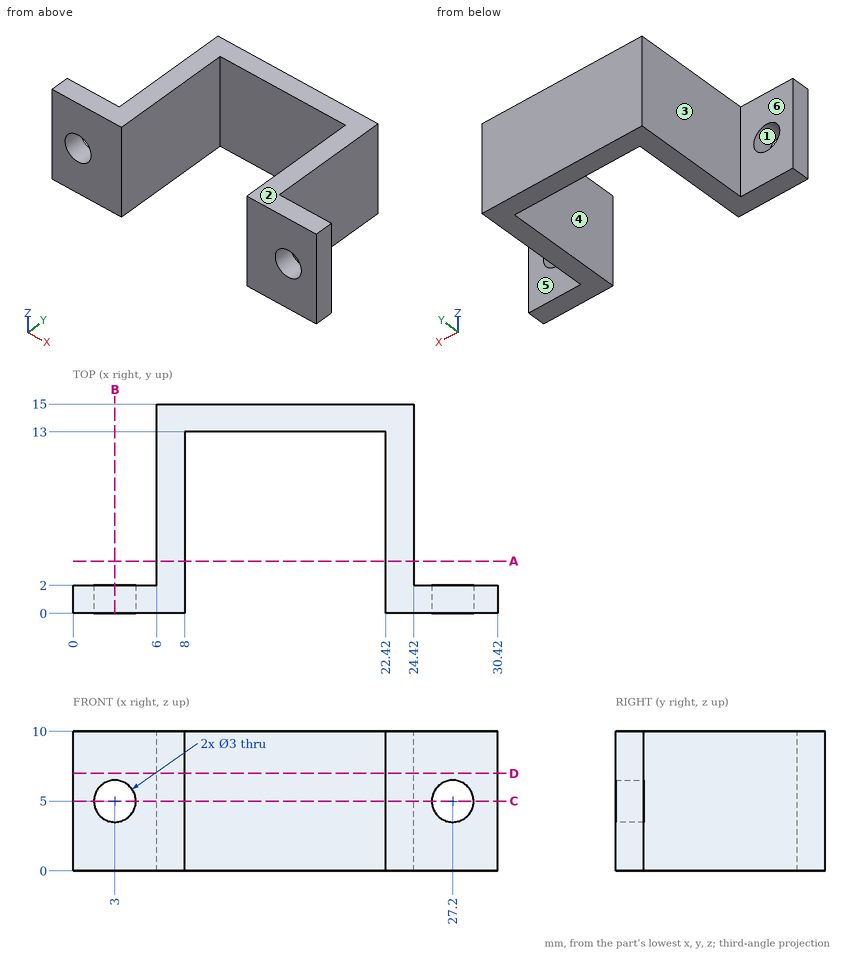
Part print with two shaded views. Sizes in mm from the minimum x, y, z corner. A direction names the side the tool comes from. Coordinates: 2 decimals unless noted, no trailing zeros. Order: outer loops, then holes, each group sorted by start corner. A loop starts at its lowest first (then second) coordinate and runs counter-clockwise, first axis right, second up.
(1) Pin check, flat tips, straight feed: pin 1 Ø1.8 at (x, z) = (3, 3) entering from +Y; pin 2 Ø5 at (y, z) = (8.5, 6.5) entering from -X; pin 3 Ø3 at (y, z) = (4, 3.5) entering from +X. Stop position of each tip, or through.
Solution:
pin 1: stops at y = 2
pin 2: stops at x = 6
pin 3: stops at x = 24.42
(2) Mould opens along Z. For the marked faces 1, 2 and 3 say: released by +Z, released by -Z, zero draft, split by the parting line, or undercut.
Solution:
face 1: undercut
face 2: released by +Z
face 3: zero draft
(3) Saw through at A-A, the plane y = 3.75. Write the cut outline in (x, z), and give its area (3 significant figures).
Solution:
outline: (6, 0) - (8, 0) - (8, 10) - (6, 10) - close; (22.42, 0) - (24.42, 0) - (24.42, 10) - (22.42, 10) - close
area: 40.0 mm2
(4) Saw through at B-B, the plane x = 3. Write the cut outline in (y, z).
Solution:
outline: (0, 0) - (2, 0) - (2, 3.5) - (0, 3.5) - close; (0, 6.5) - (2, 6.5) - (2, 10) - (0, 10) - close
(5) Saw through at D-D, the plane z = 7. Write the cut outline in (x, y), and give its area (3 significant figures).
Solution:
outline: (0, 0) - (8, 0) - (8, 13) - (22.42, 13) - (22.42, 0) - (30.42, 0) - (30.42, 2) - (24.42, 2) - (24.42, 15) - (6, 15) - (6, 2) - (0, 2) - close
area: 113 mm2
(6) Saw through at C-C, the plane z = 5. Write the cut outline in (x, y).
Solution:
outline: (0, 0) - (1.5, 0) - (1.5, 2) - (0, 2) - close; (4.5, 0) - (8, 0) - (8, 13) - (22.42, 13) - (22.42, 0) - (25.7, 0) - (25.7, 2) - (24.42, 2) - (24.42, 15) - (6, 15) - (6, 2) - (4.5, 2) - close; (28.7, 0) - (30.42, 0) - (30.42, 2) - (28.7, 2) - close
(7) Which spindle directions (+Z, -Z, +X, -X, +Y, -Y) get a long thin tool onto all of the face, cutting with end or side? Do the marked faces 4, 5 and 6. Say none if no direction does.
Solution:
face 4: +Z, -Z, -Y
face 5: +Z, -Z, +X, +Y
face 6: +Z, -Z, -X, +Y
(8) Drill centre lines: L1, parallel to X at y = 0.6, z = 5; L2, parallel to X at y = 7.5, z = 7.25; L3, parallel to X at y = 1.75, z = 6. Where is each one in solid material? Low to high.
Solution:
L1: x = 0 to 1.5, 4.5 to 8, 22.42 to 25.7, 28.7 to 30.42
L2: x = 6 to 8, 22.42 to 24.42
L3: x = 0 to 1.88, 4.12 to 8, 22.42 to 26.08, 28.32 to 30.42
